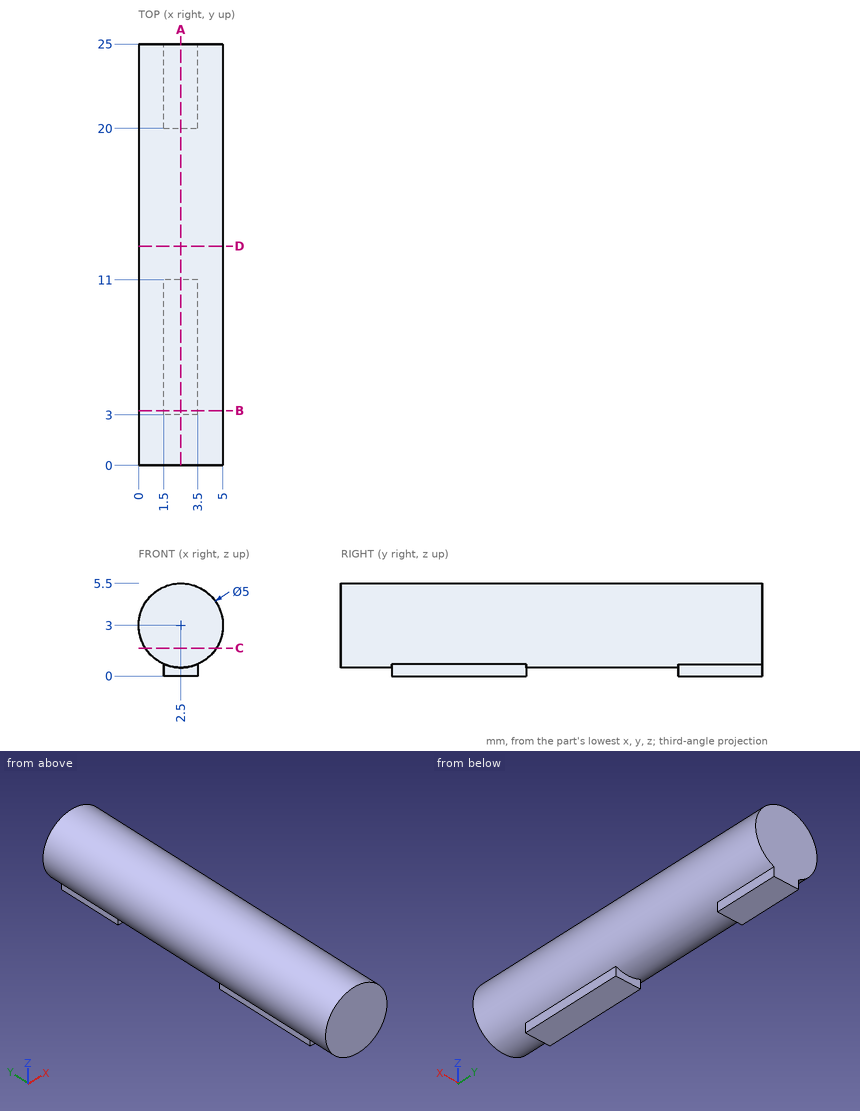
Answer from the drawing. Dimensions are ordinates in mm from the lowest x, y and z of the part. Coordinates: 2 decimals unless noted, no trailing zeros. Order: outer loops, then holes, each group sorted by start corner. A loop starts at its lowest first (then second) coordinate and runs counter-clockwise, first axis right, second up. Notation, with made-up numbers: (5, -16) - (45, -16) arc R13 cw to (45, -4) - close; hole circle Ø7 at (79.5, -5). An arc over 180 degrees is marked (long way). Answer as a JSON object with one key per item and string values. Group by question number.
Item 1: Section A-A (x = 2.5) is taken. Give the vertices of the cut face in (y, z).
Item 2: Section C-C (z = 1.65) is taken. Give the vertices of the cut face in (x, y), plus the area to 3 significant figures.
Item 3: Section D-D (y = 13) is taken. Give the vertices of the cut face in (x, z).
Item 4: Flat-ended cylindrical pins translate along their axes: P1, Ø0.8, axis at y = 6.5, z = 0, coming from the -X side; P2, Ø0.6, axis at x = 2, z = 0, coming from the -Y side. Find the tip coordinate at first contact, or state that the pin passes through.
Item 5: Section B-B (y = 3.25) is taken. Give the vertices of the cut face in (x, z).
Item 6: Consider probe 1 along Z at (x, y) = (2.55, 15.5); probe 2 along X at (y, z) = (10, 3.3); probe 3 along Z at (x, y) = (3.6, 22) (3 decimals). Determine where each line is inside the solid, lowest interval first. Write a range as from..to.
Results are:
{
 "1": {"outline": "(0, 0.5) - (3, 0.5) - (3, 0) - (11, 0) - (11, 0.5) - (20, 0.5) - (20, 0) - (25, 0) - (25, 5.5) - (0, 5.5) - close"},
 "2": {"outline": "(0.4, 0) - (4.6, 0) - (4.6, 25) - (0.4, 25) - close", "area": "105 mm^2"},
 "3": {"outline": "circle Ø5 at (2.5, 3)"},
 "4": {"P1": "stops at x = 1.5", "P2": "stops at y = 3"},
 "5": {"outline": "(1.5, 0) - (3.5, 0) - (3.5, 0.71) arc R2.5 ccw (long way) to (1.5, 0.71) - close"},
 "6": {"probe 1": "z = 0.5..5.5", "probe 2": "x = 0.02..4.98", "probe 3": "z = 0.755..5.245"}
}
